```python
from build123d import *

# Parameters (mm, degrees)
SKETCH_R      = 48.5
SKETCH_R_2    = 42
PAD_DEPTH     = 3
SKETCH001_R   = 45.5
SKETCH001_R_2 = 42
PAD001_DEPTH  = 5.5
CHAMFER_SIZE  = 1
SKETCH002_R   = 5
POCKET_DEPTH  = 5.501


with BuildPart() as part:
    # Sketch → Pad (new body)
    with BuildSketch(Plane.XY):
        Circle(SKETCH_R)
        Circle(SKETCH_R_2, mode=Mode.SUBTRACT)
    extrude(amount=PAD_DEPTH)

    # Sketch001 (on Face4 of Pad) → Pad001 (join)
    with BuildSketch(Plane.XY.offset(3)):
        Circle(SKETCH001_R)
        Circle(SKETCH001_R_2, mode=Mode.SUBTRACT)
    extrude(amount=PAD001_DEPTH)

    # Chamfer
    chamfer_edges = [part.edges().sort_by_distance(p)[0] for p in [
        (-42, 0, 8.5),
    ]]
    chamfer(chamfer_edges, length=CHAMFER_SIZE)

    # Sketch002 → Pocket (cut, through all)
    with BuildSketch(Plane.XY.offset(3)):
        with Locations((31.496593, 37.536178)):
            Circle(SKETCH002_R)
        with Locations((48.25558, 8.508761)):
            Circle(SKETCH002_R)
        with Locations((42.435245, -24.5)):
            Circle(SKETCH002_R)
        with Locations((16.758987, -46.044938)):
            Circle(SKETCH002_R)
        with Locations((-16.758987, -46.044938)):
            Circle(SKETCH002_R)
        with Locations((-42.435245, -24.5)):
            Circle(SKETCH002_R)
        with Locations((-48.25558, 8.508761)):
            Circle(SKETCH002_R)
        with Locations((-31.496593, 37.536178)):
            Circle(SKETCH002_R)
        with Locations((0, 49)):
            Circle(SKETCH002_R)
    extrude(amount=POCKET_DEPTH, mode=Mode.SUBTRACT)


solid = part.part
```
Source: CAD feature listing. Evaluate the final solid. Frame: model axes, mm. A direction names the side the tool comes from. Give positions to 0.01 mm unless a question says otherwise; leave off trailing zeros. Loops run counter-clockwise (first coordinate to the right, second up) from the corner with the lowest first, then second, coordinate; pieces in that order, holes last. Notation, with made-up numbers: (-1.5, -35.75) -> (18.5, -35.75) arc R18 cw to (18.5, -10.75) -> close; hole circle Ø8 at (-15, 26). An arc over 180 degrees is marked (long way). Use a Markdown table: item, result. Add a question column.
(1) Pull-direction query (Y, two-part tool) for faces 5 (the face through (28.24, 33.74, 5.71)), 6 (the face through (-43.34, 7.59, 5.71)), 7 (the face through (29.11, -34.97, 5.71)); classes: +Y half, -Y half, draft (parallel to the pull), parting line (faces both ways), or undercut.
(2) Ray query, line 1 (Y direction, x = 0, z = 2.5); line 2 (X direction, y = -1, z = 5); line 3 (Y direction, x = 26.5, z = 6.5). Return the intervals inside material, ascending.
(3) Section query C-C (z = 5.75). Output: boundary loops of the cut face in (x, y).
(4) Section query B-B (x = 0). Output: boundary loops of the cut face in (y, z).
(5) Section query A-A (y = 0). Output: boundary loops of the cut face in (x, z).
(6) Access query for faces 1 (the face through (15.725, 42.696, 5.712)), 2 (the face through (43.323, 7.693, 5.712)), 3 (the face through (0, 44, 6)), 4 (the face through (-0.2, -45.5, 5.7)). Directions: +Z, -Z, +X, -X, +Y, -Y. A direction counts if a zero-diameter tool reaches every point of the face in a straight line with its end or side. Return the directions, or none.
(7) First-contact query: pin 1 Ø1 at (x, z) = (15, 2) entering from +Y; pin 2 Ø5 at (y, z) = (6, 6) entering from -X; pin 3 Ø12 at (x, y) = (33, -38.5) entering from +Z; pin 4 Ø3 at (y, z) = (-2.5, 6) entering from -X. Flat tips, straight axial feed; report the tip coordinate or a pass-through.
Checked values:
| question | item | result |
|---|---|---|
| 1 | face 5 | +Y half |
| 1 | face 6 | undercut |
| 1 | face 7 | -Y half |
| 2 | line 1 | -48.5 to -42, 42 to 48.5 |
| 2 | line 2 | -45.49 to -41.99, 41.99 to 45.49 |
| 2 | line 3 | -36.99 to -32.58, 32.58 to 36.99 |
| 3 | outline | (-45.28, 4.49) arc R45.5 ccw to (-41.01, -19.71) arc R5 cw to (-37.57, -25.66) arc R45.5 ccw to (-18.75, -41.46) arc R5 cw to (-12.29, -43.81) arc R45.5 ccw to (12.29, -43.81) arc R5 cw to (18.75, -41.46) arc R45.5 ccw to (37.57, -25.66) arc R5 cw to (41.01, -19.71) arc R45.5 ccw to (45.28, 4.49) arc R5 cw to (44.08, 11.26) arc R45.5 ccw to (31.8, 32.55) arc R5 cw to (26.53, 36.97) arc R45.5 ccw to (3.44, 45.37) arc R5 cw to (-3.44, 45.37) arc R45.5 ccw to (-26.53, 36.97) arc R5 cw to (-31.8, 32.55) arc R45.5 ccw to (-44.08, 11.26) arc R5 cw to start; hole circle Ø84 at (0, 0) |
| 4 | outline | (-48.5, 0) -> (-42, 0) -> (-42, 7.5) -> (-43, 8.5) -> (-45.5, 8.5) -> (-45.5, 3) -> (-48.5, 3) -> close; (42, 0) -> (48.5, 0) -> (48.5, 3) -> (44, 3) -> (44, 8.5) -> (43, 8.5) -> (42, 7.5) -> close |
| 5 | outline | (-48.5, 0) -> (-42, 0) -> (-42, 7.5) -> (-43, 8.5) -> (-45.5, 8.5) -> (-45.5, 3) -> (-48.5, 3) -> close; (42, 0) -> (48.5, 0) -> (48.5, 3) -> (45.5, 3) -> (45.5, 8.5) -> (43, 8.5) -> (42, 7.5) -> close |
| 6 | face 1 | +Z, +X, +Y |
| 6 | face 2 | +Z, +X |
| 6 | face 3 | +Z, +Y |
| 6 | face 4 | +Z, -Y |
| 7 | pin 1 | y = 46.28 |
| 7 | pin 2 | x = -45.37 |
| 7 | pin 3 | z = 8.5 |
| 7 | pin 4 | x = -45.49 |
